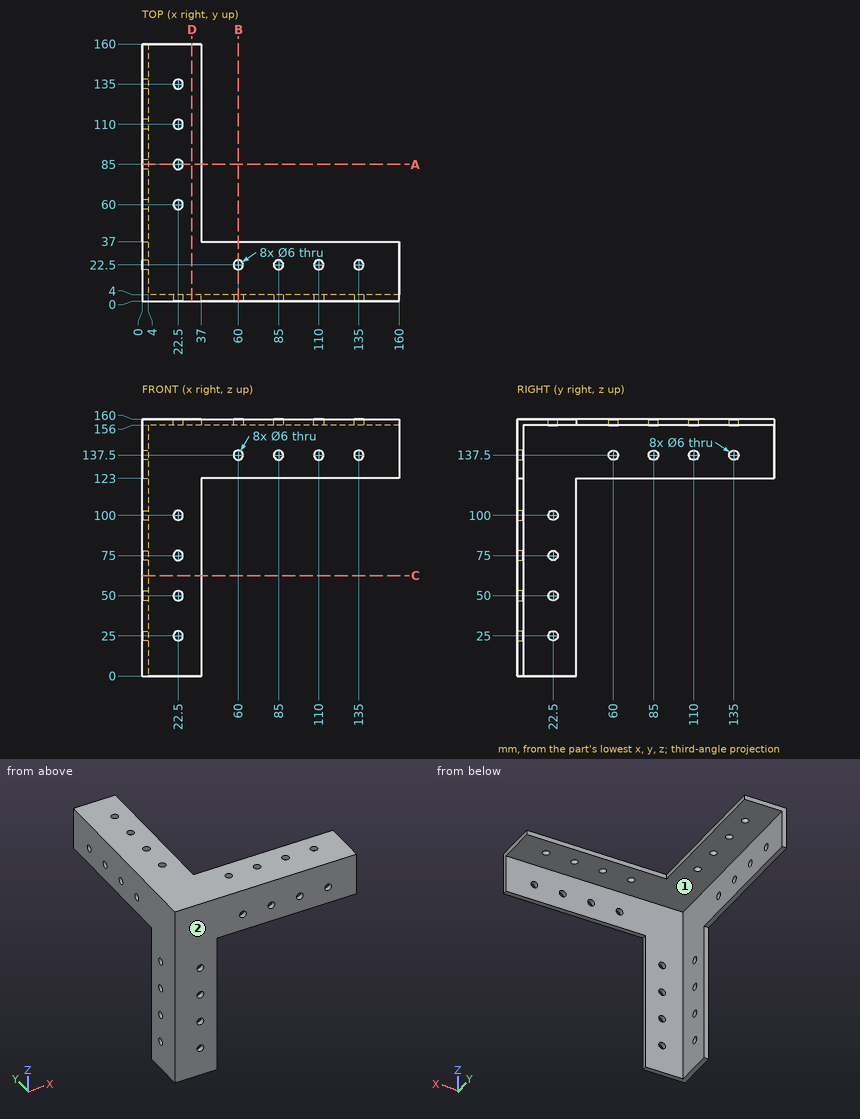
For this review, use the dimensioned drawing (mm, ordinates from the lowest corner) and the shaded views. A direction names the side the tool comes from. Give positions to 0.01 mm unless a question says otherwise; leave off trailing zeros. Write each loop counter-clockwise with the first axis right and the second up, starting at its lowest first coordinate (ties: lowest second). Pieces come first, ordered by that corner, then holes. Notation, with made-up numbers: M 41.5,-10 L 50.5,-10 A35 ccw 50.5,22 Z; hole C 13.25,60 d1. An arc over 180 degrees is marked long. Answer as a JSON object with one key per item and string values. Group by question number.
1) For line 1 along Z through (x, y) = (22, 2); line 2 along X through (y, z) = (1.2, 137.5), list the stretches that pass through material, from the lowest coordinate up.
2) We need section D-D (x = 31). Give the boundary of the cut face in (y, z), and give its area (3 significant figures).
3) We need section A-A (y = 85). Give the boundary of the cut face in (x, z), and give its area (3 significant figures).
4) Tool access review of the marked faces 1 and 2: name each direction out of +Z, -Z, +X, -X, +Y, -Y from which nothing blocks a thin tool from reaching the whole face with its end or side.
5) Clearance check with flat-ended pins moving along their axes: pin 1 Ø5.5 at (x, y) = (110, 22.5) entering from +Z; pin 2 Ø1.2 at (x, y) = (2, 94) entering from -Z; pin 3 Ø8 at (y, z) = (110, 137.5) entering from +X; pin 4 Ø8 at (x, z) = (22, 84) entering from +Y. State where each tip first meets the part, or that it passes through.
6) We need section C-C (z = 62.5). Give the boundary of the cut face in (x, y).
Answer key:
{
 "1": {"line 1": "z = 0 to 22.04, 27.96 to 47.04, 52.96 to 72.04, 77.96 to 97.04, 102.96 to 160", "line 2": "x = 0 to 57, 63 to 82, 88 to 107, 113 to 132, 138 to 160"},
 "2": {"outline": "M 0,0 L 4,0 L 4,156 L 160,156 L 160,160 L 0,160 Z", "area": "1,260 mm²"},
 "3": {"outline": "M 0,123 L 4,123 L 4,134.5 L 0,134.5 Z; M 0,140.5 L 4,140.5 L 4,156 L 19.5,156 L 19.5,160 L 0,160 Z; M 25.5,156 L 37,156 L 37,160 L 25.5,160 Z", "area": "232 mm²"},
 "4": {"face 1": "-Z, +X, +Y", "face 2": "+Z, -Z, +X, -X, -Y"},
 "5": {"pin 1": "passes through", "pin 2": "stops at z = 123", "pin 3": "stops at x = 4", "pin 4": "stops at y = 4"},
 "6": {"outline": "M 0,0 L 37,0 L 37,4 L 4,4 L 4,37 L 0,37 Z"}
}
